from build123d import *

# Parameters (mm, degrees)
SKETCH_1_R          = 7.9
SKETCH_1_R_2        = 5
EXTRUDE_1_DEPTH     = 2.7
CUT_EXTRUDE_1_DEPTH = 10


with BuildPart() as part:
    # 草图1 → 凸台-拉伸1 (new body)
    with BuildSketch(Plane.XY):
        with Locations(Location((0, 0, 0), (0, 0, 180))):
            Circle(SKETCH_1_R)
        with Locations(Location((0, 0, 0), (0, 0, 180))):
            Circle(SKETCH_1_R_2, mode=Mode.SUBTRACT)
    extrude(amount=EXTRUDE_1_DEPTH)

    # 草图2 → 切除-拉伸1 (cut)
    with BuildSketch(Plane.XY.offset(2.7)):
        Polygon((0, 0), (8.171451681, 4.033670186), (8.171451681, 3.587869008), align=None)
    extrude(amount=-CUT_EXTRUDE_1_DEPTH, mode=Mode.SUBTRACT)


solid = part.part
Verification items for the finished model (mm, model axes). A direction names the side the tool comes from. Coordinates: 2 decimals unless noted, no trailing zeros. Order: outer loops, then holes, each group sorted by start corner. A loop starts at its lowest first (then second) coordinate and runs counter-clockwise, first axis right, second up. Notation, with made-up numbers: M 79.25,-39.5 L 94.25,-39.5 A19 ccw 94.25,-17.5 Z; hole C 66.5,80 d9. An arc over 180 degrees is marked long. Write each question's results on one line, items separated by ' | '.
1) Scan lines: line 1 along Y through (x, z) = (0, 0.85); line 2 along Y through (x, z) = (5.25, 2.5); line 3 along X through (y, z) = (-2.25, 2.35). Record each from-to range of solid material in increasing order. Write a range as [from, to].
Solved:
line 1: y = [-7.9, -5], [5, 7.9] | line 2: y = [-5.9, 2.31], [2.59, 5.9] | line 3: x = [-7.57, -4.47], [4.47, 7.57]
2) Section check D-D on y = -6.5. Record the cut outline in (x, z).
Solved:
outline: M -4.49,0 L 4.49,0 L 4.49,2.7 L -4.49,2.7 Z
3) Release check for a two-part mould opening along X. For faces 3 (the face through (0.1, 5.2, 0)), 4 (the face through (5.77, 2.85, 1.37)) record: pulls with the +X half, pulls with the -X half, needs draft (parallel to the pull), parting line crosses it, or undercut.
Solved:
face 3: needs draft | face 4: undercut
4) Section check C-C on z = 0.75. Record the cut outline in (x, y), plus the area to 3 significant figures.
Solved:
outline: M 4.48,2.21 L 7.08,3.5 A7.9 ccw long 7.23,3.18 L 4.58,2.01 A5 cw long Z | area: 117 mm²
5) Access from +Z, -Z, +X, -X, +Y, -Y to the whole of each face (thin tool, end or side, straight path). Record for faces 1 (the face through (0.1, 5.2, 2.7)), 2 (the face through (5.92, 2.6, 1.37)).
Solved:
face 1: +Z, +X, -X, +Y, -Y | face 2: +Z, -Z
6) Section check A-A on x = 0. Record the cut outline in (y, z).
Solved:
outline: M -7.9,0 L -5,0 L -5,2.7 L -7.9,2.7 Z; M 5,0 L 7.9,0 L 7.9,2.7 L 5,2.7 Z
7) Gauge pin test, flat ends, axial feed: pin 1 Ø1 at (y, z) = (3.5, 0.5) entering from +X; pin 2 Ø1 at (x, z) = (1, 0.5) entering from +Y; pin 3 Ø1.5 at (y, z) = (5.5, 1) entering from -X. Record the tip position at first contact, or that the pin passes through.
Solved:
pin 1: stops at x = 7.31 | pin 2: stops at y = 7.88 | pin 3: stops at x = -6.31
8) Section check B-B on y = -2.5. Record the cut outline in (x, z).
Solved:
outline: M -7.49,0 L -4.33,0 L -4.33,2.7 L -7.49,2.7 Z; M 4.33,0 L 7.49,0 L 7.49,2.7 L 4.33,2.7 Z
